```python
from build123d import *

# Parameters (mm, degrees)
PAD_DEPTH    = 0.25
PAD001_DEPTH = 0.5
SKETCH003_R  = 0.15
PAD002_DEPTH = 0.5


with BuildPart() as part:
    # Sketch → Pad (new body, symmetric)
    with BuildSketch(Plane.XY):
        with BuildLine():
            Line((-0.375, 0), (0, 0))
            Line((0, 0), (0.375, 0))
            ThreePointArc((0.375, 0), (9.051962, -20.948038), (30, -29.625))
            ThreePointArc((30.000004, -30.375), (30.375, -29.999998), (30, -29.625))
            ThreePointArc((-0.375, 0), (8.521633, -21.47837), (30.000004, -30.375))
        make_face()
    extrude(amount=PAD_DEPTH, both=True)

    # Sketch002 → Pad001 (join)
    with BuildSketch(Plane.XZ):
        with BuildLine():
            ThreePointArc((-1.25, 0.75), (-1.426777, 0.676777), (-1.5, 0.5))
            Line((-1.5, -0.5), (-1.5, 0.5))
            ThreePointArc((-1.5, -0.5), (-1.426777, -0.676777), (-1.25, -0.75))
            Line((1.25, -0.75), (-1.25, -0.75))
            ThreePointArc((1.25, -0.75), (1.426777, -0.676777), (1.5, -0.5))
            Line((1.5, 0.5), (1.5, -0.5))
            ThreePointArc((1.5, 0.5), (1.426777, 0.676777), (1.25, 0.75))
            Line((-1.25, 0.75), (1.25, 0.75))
        make_face()
    extrude(amount=PAD001_DEPTH)

    # Sketch003 (on DatumPlane) → Pad002 (join)
    with BuildSketch(Plane(origin=(30, -30, 0.25), x_dir=(1, 0, 0), z_dir=(0, 0, 1))):
        Circle(SKETCH003_R)
    extrude(amount=PAD002_DEPTH)


solid = part.part
```
Work out the finished part from the listing and answer in its coordinate system (mm). Give positions to 0.01 mm unless a question says otherwise; leave off trailing zeros. Order: outer loops, then holes, each group sorted by start corner. A loop starts at its lowest first (then second) coordinate and runs counter-clockwise, first axis right, second up. Notation, with made-up numbers: (7.25, 33.5) -> (43.25, 33.5) arc R23 cw to (43.25, 43.5) -> close; hole circle Ø11 at (4, 86.25). An arc over 180 degrees is marked (long way). Answer as CSV lines item,"result". Start each with the question number.
(1) Section A-A, the plane z = 0 is taken. Write down the section's boundary in (x, y) (3 decimals), plus the area to 3 significant figures.
(2) Consider line 1 along X through (y, z) = (-4.5, -0.15); line 2 along X through (y, z) = (-26, 0.05); line 3 along Y through (x, z) = (5, 0.2). Determine where each line is inside the solid, lowest interval first.
(3) For a pull along Y with two mould halves and no side action, classify faces 1 (the flat face through (9.4, -22, 0.25)), 2 (the cylindrical face through (8.465, -21.421, 0.004)), 3 (the flat face through (0, 0, 0)), 4 (the cylindrical face through (9.001, -20.897, 0.004)) as released by +Y, released by -Y, zero draft, split by the parting line, or undercut.
(4) Section B-B, the plane x = 28.5 is taken. Write down the section's boundary in (y, z), plus the area to 3 significant figures.
(5) Each of these flat-tipped pins is pushed along its axis until it touches: pin 1 Ø1 at (x, y) = (8, -19) entering from +Z; pin 2 Ø0.6 at (y, z) = (0, 0) entering from +X. Where does it stop, or does it pass through?
(6) Section C-C, the plane y = -17 is taken. Write down the section's boundary in (x, z), plus the area to 3 significant figures.
Entries:
1,outline,"(-1.5, -0.5) -> (-0.371, -0.5) arc R30.375 ccw to (30, -30.375) arc R0.375 ccw to (30, -29.625) arc R29.625 cw to (0.379, -0.5) -> (1.5, -0.5) -> (1.5, 0) -> (-1.5, 0) -> close"
1,area,"36.7 mm²"
2,line 1,"-0.04 to 0.72"
2,line 2,"14.3 to 15.8"
2,line 3,"-17.25 to -15.89"
3,face 1,"zero draft"
3,face 2,"released by -Y"
3,face 3,"released by +Y"
3,face 4,"undercut"
4,outline,"(-30.34, -0.25) -> (-29.59, -0.25) -> (-29.59, 0.25) -> (-30.34, 0.25) -> close"
4,area,"0.375 mm²"
5,pin 1,"through"
5,pin 2,"x = 1.5"
6,outline,"(4.83, -0.25) -> (5.74, -0.25) -> (5.74, 0.25) -> (4.83, 0.25) -> close"
6,area,"0.455 mm²"
